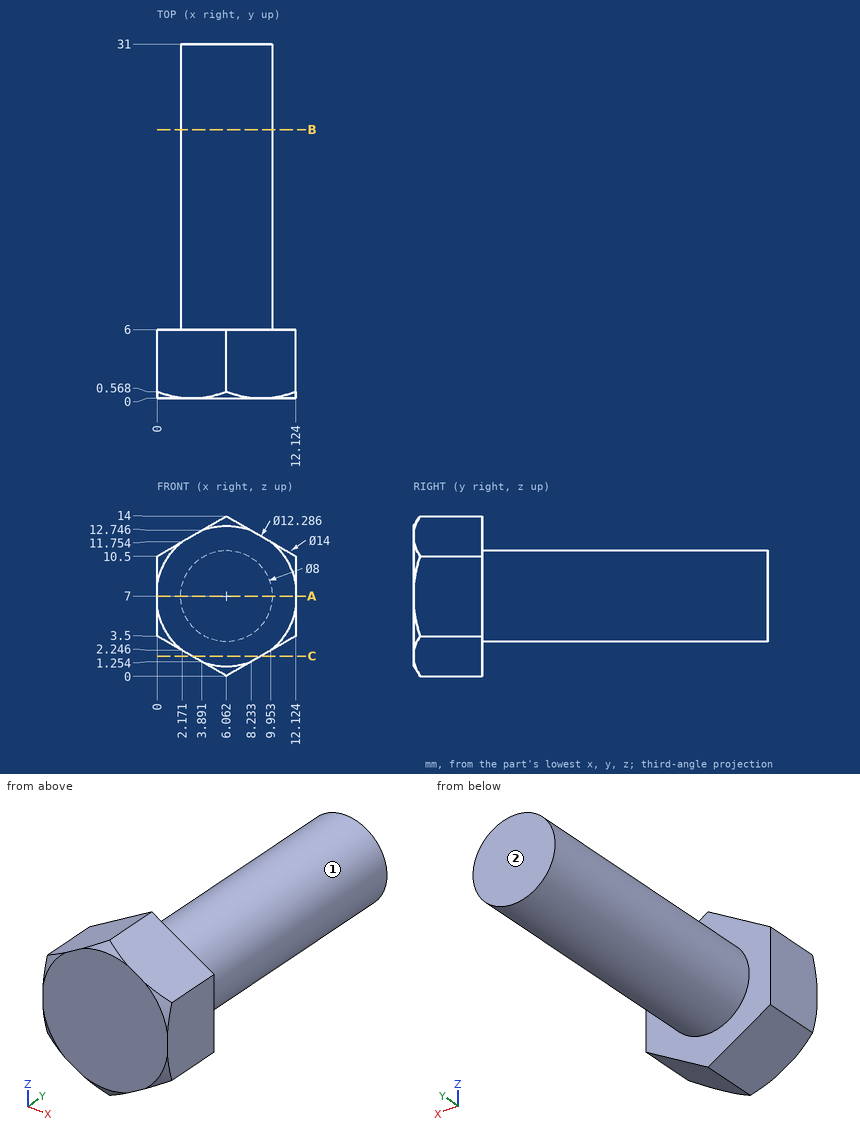
Drawing for the job (mm, zero at the part's lowest x, y, z). A direction names the side the tool comes from. Give positions to 0.01 mm unless a question says otherwise; leave off trailing zeros. Loops run counter-clockwise (first coordinate to the right, second up) from the corner with the lowest first, then second, coordinate; pieces in that order, holes last. Notation, with made-up numbers: (-36, 2.25) - (18, 2.25) arc R24 cw to (18, 24.25) - close; hole circle Ø5 at (30, 60.25). An arc over 180 degrees is marked (long way). Write item = value, one per line. Start each with the question number.
1) Probe probe 1 along Y at (x, z) = (1.25, 8.25); probe 2 along Z at (x, y) = (8, 10); probe 3 along Z at (x, y) = (5.5, 29). List the from-to ranges inside material, lowest first. Write a range as from..to.
2) Band-saw the part on B-B on y = 23.5. Give the cut face in (x, z).
3) Band-saw the part on A-A on z = 7. Give the cut face in (x, y) (1 decimal), plus the area to 3 significant figures.
4) Band-saw the part on C-C on z = 1.75. Give the cut face in (x, y).
5) Drop flat-ended pins along their axis: pin 1 Ø6 at (y, z) = (19.5, 10.5) entering from -X; pin 2 Ø5 at (x, y) = (10.5, 20.5) entering from +Z; pin 3 Ø4 at (y, z) = (27.5, 9) entering from +X; pin 4 Ø8 at (y, z) = (8, 12) entering from -X. Give the stop position or say it passes through.
6) Tool access for the marked faces 1 and 2: list every direction of +Z, -Z, +X, -X, +Y, -Y with a clear straight run to the whole face (end or side of a thin tool).
Final values:
q1.probe_1 = 0..6
q1.probe_2 = 3.5..10.5
q1.probe_3 = 3.04..10.96
q2.outline = circle Ø8 at (6.06, 7)
q3.outline = (0, 0) - (12.1, 0) - (12.1, 6) - (10.1, 6) - (10.1, 31) - (2.1, 31) - (2.1, 6) - (0, 6) - close
q3.area = 273 mm²
q4.outline = (3.03, 0) - (9.09, 0) - (9.09, 6) - (3.03, 6) - close
q5.pin_1 = 2.09
q5.pin_2 = 10.5
q5.pin_3 = 10.06
q5.pin_4 = 0
q6.face_1 = +Y
q6.face_2 = +Z, -Z, +X, -X, +Y
